```python
from build123d import *

# Parameters (mm, degrees)
SKETCH1_W           = 25
SKETCH1_H           = 25
SKETCH1_R           = 12
SKETCH1_R_2         = 1.4
BOSS_EXTRUDE1_DEPTH = 10
FILLET1_R           = 2.5
SKETCH2_R           = 8
BOSS_EXTRUDE2_DEPTH = 10
SKETCH3_W           = 1.5
SKETCH3_H           = 4.535233839
BOSS_EXTRUDE3_DEPTH = 10


with BuildPart() as part:
    # Sketch1 → Boss-Extrude1 (new body)
    with BuildSketch(Plane.XY):
        with Locations((12.5, 12.5)):
            Rectangle(SKETCH1_W, SKETCH1_H)
        with Locations((12.5, 12.5)):
            Circle(SKETCH1_R, mode=Mode.SUBTRACT)
        with Locations((2.5, 22.5)):
            Circle(SKETCH1_R_2, mode=Mode.SUBTRACT)
        with Locations((2.5, 2.5)):
            Circle(SKETCH1_R_2, mode=Mode.SUBTRACT)
        with Locations((22.5, 22.5)):
            Circle(SKETCH1_R_2, mode=Mode.SUBTRACT)
    extrude(amount=BOSS_EXTRUDE1_DEPTH)

    # Fillet1
    fillet1_edges = [part.edges().sort_by_distance(p)[0] for p in [
        (0, 25, 5),
        (25, 25, 5),
        (25, 0, 5),
        (0, 0, 5),
    ]]
    fillet(fillet1_edges, radius=FILLET1_R)



with BuildPart() as body_2:
    # Sketch2 → Boss-Extrude2 (new body)
    with BuildSketch(Plane.XY.offset(10)):
        with Locations((12.5, 12.5)):
            Circle(SKETCH2_R)
    extrude(amount=-BOSS_EXTRUDE2_DEPTH)


with BuildPart() as part_1:
    add(part.part)

    add(body_2.part)  # Boss-Extrude3 merges body 2
    # Sketch3 → Boss-Extrude3 (add)
    with BuildSketch(Plane.XY.offset(10)):
        with Locations((12.5, 22.732383081)):
            Rectangle(SKETCH3_W, SKETCH3_H)
        Polygon((23.700317547, 6.899519053), (22.950317547, 5.600480947), (19.022689831, 7.868097867), (19.772689831, 9.167135972), align=None)
        Polygon((2.049682453, 5.600480947), (1.299682453, 6.899519053), (5.227310169, 9.167135972), (5.977310169, 7.868097867), align=None)
    extrude(amount=-BOSS_EXTRUDE3_DEPTH)


solid = part_1.part
```
Design review of the part built by this model. Coordinates are the model's own, in mm. A direction names the side the tool comes from. Round coordinates to 2 decimals unless told otherwise and drop trailing zeros. Order: outer loops, then holes, each group sorted by start corner. A loop starts at its lowest first (then second) coordinate and runs counter-clockwise, first axis right, second up. Notation, with made-up numbers: M 12.25,14 L 55.25,14 A25 ccw 55.25,27 Z; hole C -37.5,-18 d9. An arc over 180 degrees is marked long. Put each result on its own line as item: value.
Q1. Consider section A-A (z = 9.25). State the section outline as (x, y) points.
Reported:
outline: M 0,2.5 A2.5 ccw 2.5,0 L 22.5,0 A2.5 ccw 25,2.5 L 25,22.5 A2.5 ccw 22.5,25 L 2.5,25 A2.5 ccw 0,22.5 Z; hole C 2.5,2.5 d2.8; hole C 2.5,22.5 d2.8; hole M 1.75,7.16 L 5.23,9.17 A8 cw 11.75,20.46 L 11.75,24.48 A12 ccw Z; hole M 2.5,5.86 A12 ccw 22.5,5.86 L 19.02,7.87 A8 cw 5.98,7.87 Z; hole M 13.25,20.46 A8 cw 19.77,9.17 L 23.25,7.16 A12 ccw 13.25,24.48 Z; hole C 22.5,22.5 d2.8
Q2. Consider section D-D (y = 21.5). State the section outline as (x, z) points.
Reported:
outline: M 0,0 L 1.52,0 L 1.52,10 L 0,10 Z; M 3.48,0 L 4.56,0 L 4.56,10 L 3.48,10 Z; M 11.75,0 L 13.25,0 L 13.25,10 L 11.75,10 Z; M 20.44,0 L 21.52,0 L 21.52,10 L 20.44,10 Z; M 23.48,0 L 25,0 L 25,10 L 23.48,10 Z
Q3. Machinability: for faces 1 (the face through (24.248, 24.287, 5.07)), 2 (the face through (12.4, 4.5, 5.1)), which of the approach directions +Z, -Z, +X, -X, +Y, -Y give a long, thin tool a straight path to every point of the face, cutting with its end or side? Answer none if there is none.
Reported:
face 1: +Z, -Z, +X, +Y
face 2: +Z, -Z
Q4. Draft analysis for pull direction X (two halves, no side actions). For faces 3 (the face through (12, 0, 5)), 4 (the face through (0.713, 0.752, 5.07)), 5 (the face through (2.19, 18.64, 4.93)), state which applies: released by +X, released by -X, zero draft, split by the parting line, or undercut.
Reported:
face 3: zero draft
face 4: released by -X
face 5: undercut
Q5. Consider section B-B (x = 15.5). State the section outline as (y, z) points.
Reported:
outline: M 0,0 L 0.88,0 L 0.88,10 L 0,10 Z; M 5.08,0 L 19.92,0 L 19.92,10 L 5.08,10 Z; M 24.12,0 L 25,0 L 25,10 L 24.12,10 Z
Q6. Consider section C-C (y = 13.5). State the section outline as (x, z) points, and give its area (3 significant figures).
Reported:
outline: M 0,0 L 0.54,0 L 0.54,10 L 0,10 Z; M 4.56,0 L 20.44,0 L 20.44,10 L 4.56,10 Z; M 24.46,0 L 25,0 L 25,10 L 24.46,10 Z
area: 170 mm²
Q7. Insertion check: pin 1 Ø4 at (x, y) = (15.5, 15.5) entering from -Z. The pin has a flat end and moves straight along its axis. Give the tip position at first contact, or say it passes through.
Reported:
pin 1: z = 0
Q8. To check wall thickness, follow line 1 (X direction, y = 12.75, z = 8.75); line 2 (X direction, y = 10.25, z = 2.5); line 3 (Y direction, x = 4, z = 3.5). State the ranges of each line that lie inside material, in increasing order.
Reported:
line 1: 0 to 0.5, 4.5 to 20.5, 24.5 to 25
line 2: 0 to 0.71, 4.82 to 20.18, 24.29 to 25
line 3: 0 to 4.03, 6.73 to 8.46, 20.97 to 25
